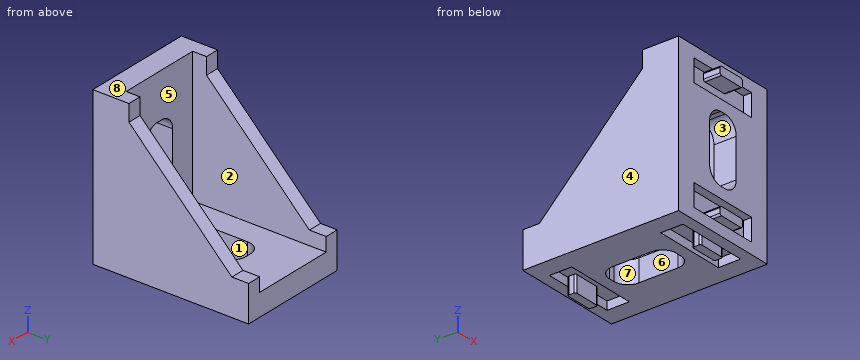
from build123d import *

# Parameters (mm, degrees)
F0_W      = 20
F0_H      = 28
F1_DEPTH  = 4
F2_W      = 20
F2_H      = 28
F3_DEPTH  = 4
F4_W      = 13
F4_H      = 4
F5_DEPTH  = 1.5
F7_DEPTH  = 3
F9_DEPTH  = 3
F11_DEPTH = 4
F12_W     = 13
F12_H     = 4
F13_DEPTH = 1.5
F15_DEPTH = 4
F17_DEPTH = 3
F19_DEPTH = 3
F21_DEPTH = 2.5
F23_DEPTH = 2.5


with BuildPart() as f1:
    # F0 (on Top) → F1 (new body)
    with BuildSketch(Plane.XY):
        with Locations((-10, 14)):
            Rectangle(F0_W, F0_H)
    extrude(amount=F1_DEPTH)

    # F2 (on Front) → F3 (join)
    with BuildSketch(Plane.XZ):
        with Locations((-10, 14)):
            Rectangle(F2_W, F2_H)
    extrude(amount=-F3_DEPTH)

    # F4 (on face) → F5 (cut)
    with BuildSketch(Plane.XZ):
        with Locations((-10, 4)):
            Rectangle(F4_W, F4_H)
        with Locations((-10, 24)):
            Rectangle(F4_W, F4_H)
    extrude(amount=-F5_DEPTH, mode=Mode.SUBTRACT)

    # F6 (on face) → F7 (join)
    with BuildSketch(Plane.XZ.offset(-1.5)):
        with BuildLine():
            Line((-7.8, 3.5), (-12.2, 3.5))
            ThreePointArc((-12.2, 3.5), (-12.4121320344, 3.4121320344), (-12.5, 3.2))
            Line((-12.5, 3.2), (-12.5, 2.3))
            ThreePointArc((-12.5, 2.3), (-12.4121320344, 2.0878679656), (-12.2, 2))
            Line((-12.2, 2), (-7.8, 2))
            ThreePointArc((-7.8, 2), (-7.5878679656, 2.0878679656), (-7.5, 2.3))
            Line((-7.5, 2.3), (-7.5, 3.2))
            ThreePointArc((-7.5, 3.2), (-7.5878679656, 3.4121320344), (-7.8, 3.5))
        make_face()
    extrude(amount=F7_DEPTH)

    # F8 (on face) → F9 (join)
    with BuildSketch(Plane.XZ.offset(-1.5)):
        with BuildLine():
            Line((-7.8, 26), (-12.2, 26))
            ThreePointArc((-12.2, 26), (-12.4121320344, 25.9121320344), (-12.5, 25.7))
            Line((-12.5, 25.7), (-12.5, 24.8))
            ThreePointArc((-12.5, 24.8), (-12.4121320344, 24.5878679656), (-12.2, 24.5))
            Line((-12.2, 24.5), (-7.8, 24.5))
            ThreePointArc((-7.8, 24.5), (-7.5878679656, 24.5878679656), (-7.5, 24.8))
            Line((-7.5, 24.8), (-7.5, 25.7))
            ThreePointArc((-7.5, 25.7), (-7.5878679656, 25.9121320344), (-7.8, 26))
        make_face()
    extrude(amount=F9_DEPTH)

    # F10 (on face) → F11 (cut)
    with BuildSketch(Plane.XZ):
        with BuildLine():
            Line((-7, 10.5), (-7, 14))
            Line((-7, 14), (-13, 14))
            Line((-13, 14), (-13, 10.5))
            ThreePointArc((-13, 10.5), (-12.267766953, 8.732233047), (-10.5, 8))
            Line((-10.5, 8), (-9.5, 8))
            ThreePointArc((-9.5, 8), (-7.732233047, 8.732233047), (-7, 10.5))
        make_face()
        with BuildLine():
            Line((-13, 14), (-7, 14))
            Line((-7, 14), (-7, 17.5))
            ThreePointArc((-7, 17.5), (-7.732233047, 19.267766953), (-9.5, 20))
            Line((-9.5, 20), (-10.5, 20))
            ThreePointArc((-10.5, 20), (-12.267766953, 19.267766953), (-13, 17.5))
            Line((-13, 17.5), (-13, 14))
        make_face()
    extrude(amount=-F11_DEPTH, mode=Mode.SUBTRACT)

    # F12 (on face) → F13 (cut)
    with BuildSketch(Plane(origin=(0, 0, 0), x_dir=(1, 0, 0), z_dir=(0, 0, -1))):
        with Locations((-10, -24)):
            Rectangle(F12_W, F12_H)
        with Locations((-10, -4)):
            Rectangle(F12_W, F12_H)
    extrude(amount=-F13_DEPTH, mode=Mode.SUBTRACT)

    # F14 (on face) → F15 (cut)
    with BuildSketch(Plane(origin=(0, 0, 0), x_dir=(1, 0, 0), z_dir=(0, 0, -1))):
        with BuildLine():
            Line((-6.9838613272, -14), (-12.9838613272, -14))
            Line((-12.9838613272, -14), (-12.9838613272, -17.5))
            ThreePointArc((-12.9838613272, -17.5), (-12.2516282801, -19.267766953), (-10.4838613272, -20))
            Line((-10.4838613272, -20), (-9.4838613272, -20))
            ThreePointArc((-9.4838613272, -20), (-7.7160943742, -19.267766953), (-6.9838613272, -17.5))
            Line((-6.9838613272, -17.5), (-6.9838613272, -14))
        make_face()
        with BuildLine():
            Line((-9.4838613272, -8), (-10.4838613272, -8))
            ThreePointArc((-10.4838613272, -8), (-12.2516282801, -8.732233047), (-12.9838613272, -10.5))
            Line((-12.9838613272, -10.5), (-12.9838613272, -14))
            Line((-12.9838613272, -14), (-6.9838613272, -14))
            Line((-6.9838613272, -14), (-6.9838613272, -10.5))
            ThreePointArc((-6.9838613272, -10.5), (-7.7160943742, -8.732233047), (-9.4838613272, -8))
        make_face()
    extrude(amount=-F15_DEPTH, mode=Mode.SUBTRACT)

    # F16 (on face) → F17 (join)
    with BuildSketch(Plane(origin=(0, 0, 1.5), x_dir=(1, 0, 0), z_dir=(0, 0, -1))):
        with BuildLine():
            Line((-7.8, -24.5), (-12.2, -24.5))
            ThreePointArc((-12.2, -24.5), (-12.4121320344, -24.5878679656), (-12.5, -24.8))
            Line((-12.5, -24.8), (-12.5, -25.7))
            ThreePointArc((-12.5, -25.7), (-12.4121320344, -25.9121320344), (-12.2, -26))
            Line((-12.2, -26), (-7.8, -26))
            ThreePointArc((-7.8, -26), (-7.5878679656, -25.9121320344), (-7.5, -25.7))
            Line((-7.5, -25.7), (-7.5, -24.8))
            ThreePointArc((-7.5, -24.8), (-7.5878679656, -24.5878679656), (-7.8, -24.5))
        make_face()
    extrude(amount=F17_DEPTH)

    # F18 (on face) → F19 (join)
    with BuildSketch(Plane(origin=(0, 0, 1.5), x_dir=(1, 0, 0), z_dir=(0, 0, -1))):
        with BuildLine():
            Line((-12.2, -3.5), (-7.8, -3.5))
            ThreePointArc((-7.8, -3.5), (-7.5878679656, -3.4121320344), (-7.5, -3.2))
            Line((-7.5, -3.2), (-7.5, -2.3))
            ThreePointArc((-7.5, -2.3), (-7.5878679656, -2.0878679656), (-7.8, -2))
            Line((-7.8, -2), (-12.2, -2))
            ThreePointArc((-12.2, -2), (-12.4121320344, -2.0878679656), (-12.5, -2.3))
            Line((-12.5, -2.3), (-12.5, -3.2))
            ThreePointArc((-12.5, -3.2), (-12.4121320344, -3.4121320344), (-12.2, -3.5))
        make_face()
    extrude(amount=F19_DEPTH)

    # F20 (on face) → F21 (join)
    with BuildSketch(Plane.YZ):
        Polygon((4, 4), (28, 4), (28, 6.5), (25, 6.5), (6.5, 25), (6.5, 28), (4, 28), align=None)
    extrude(amount=-F21_DEPTH)

    # F22 (on face) → F23 (join)
    with BuildSketch(Plane(origin=(-20, 0, 0), x_dir=(0, -1, 0), z_dir=(-1, 0, 0))):
        Polygon((-4, 4), (-4, 28), (-6.5, 28), (-6.5, 25), (-25, 6.5), (-28, 6.5), (-28, 4), align=None)
    extrude(amount=-F23_DEPTH)


solid = f1.part
Read the model definition and answer for the solid it produces. Units are mm, in the model's axes. Face numbers are marked on the shaded views. A direction names the side the tool comes from. Round coordinates to 2 decimals unless told otherwise and drop trailing zeros. Loops run counter-clockwise (first coordinate to the right, second up) from the corner with the lowest first, then second, coordinate; pieces in that order, holes last.
Q1. Determine the mould class of the marked faces 5, 6, 7 and 8 for opening direction Y: released by +Y, released by -Y, zero draft, split by the parting line, or undercut.
Q2. Consider probe 1 along X at (y, z) = (3, 1); probe 2 along X at (y, z) = (23.5, 6); probe 3 along Y at (x, z) = (-8.75, 1.25). Determine where each line is inside the solid, lowest interval first.
Q3. Each of these flat-tipped pins is pushed along its axis until it touches: pin 1 (10 mm diameter, centred on x = -10.5, z = 15, fed in from -Y); pin 2 (5 mm diameter, centred on x = -12, y = 7.5, fed in from +Z); pin 3 (2 mm diameter, centred on x = -12.5, z = 23.5, fed in from -Y). Where does it stop, or does it pass through?
Q4. Section D-D on z = 24 is taken. Write down the section's boundary in (x, y), and give its area (3 significant figures).
Q5. Which of the six approach directions +Z, -Z, +X, -X, +Y, -Y give full straight-line access (tool end or side, diameter ignored) to the marked faces 1, 2, 3 and 4?
Q6. Section A-A on y = 16 is taken. Write down the section's boundary in (x, z).
Q7. Section C-C on y = 2.75 is taken. Write down the section's boundary in (x, z).
Q8. Section B-B on z = 12.25 is taken. Write down the section's boundary in (x, y), and give its area (3 significant figures).
Output:
1. face 5: released by +Y
1. face 6: undercut
1. face 7: undercut
1. face 8: zero draft
2. probe 1: x = -20 to -16.5, -12.5 to -7.5, -3.5 to 0
2. probe 2: x = -20 to -17.5, -2.5 to 0
2. probe 3: y = 0 to 3.5, 6 to 8.11, 19.89 to 22, 24.5 to 28
3. pin 1: stops at y = 0
3. pin 2: stops at z = 4
3. pin 3: stops at y = 1.5
4. outline: (-20, 0) - (-16.5, 0) - (-16.5, 1.5) - (-3.5, 1.5) - (-3.5, 0) - (0, 0) - (0, 7.5) - (-2.5, 7.5) - (-2.5, 4) - (-17.5, 4) - (-17.5, 7.5) - (-20, 7.5) - close
4. area: 78.0 mm2
5. face 1: +Z, -Z
5. face 2: +Z, +Y
5. face 3: +Y, -Y
5. face 4: +Z, -Z, -X, +Y, -Y
6. outline: (-20, 0) - (-12.98, 0) - (-12.98, 4) - (-17.5, 4) - (-17.5, 15.5) - (-20, 15.5) - close; (-6.98, 0) - (0, 0) - (0, 15.5) - (-2.5, 15.5) - (-2.5, 4) - (-6.98, 4) - close
7. outline: (-20, 0) - (-16.5, 0) - (-16.5, 1.5) - (-12.5, 1.5) - (-12.5, -1.5) - (-7.5, -1.5) - (-7.5, 1.5) - (-3.5, 1.5) - (-3.5, 0) - (0, 0) - (0, 28) - (-20, 28) - close; hole (-13, 10.5) arc R2.5 ccw to (-10.5, 8) - (-9.5, 8) arc R2.5 ccw to (-7, 10.5) - (-7, 17.5) arc R2.5 ccw to (-9.5, 20) - (-10.5, 20) arc R2.5 ccw to (-13, 17.5) - close
8. outline: (-20, 0) - (-13, 0) - (-13, 4) - (-17.5, 4) - (-17.5, 19.25) - (-20, 19.25) - close; (-7, 0) - (0, 0) - (0, 19.25) - (-2.5, 19.25) - (-2.5, 4) - (-7, 4) - close
8. area: 132 mm2
